from build123d import *

# Parameters (mm, degrees)
F0_R          = 3.85802972
F2_DEPTH      = 3.81
F2_DEPTH_BACK = 3.81
F4_D          = 3.2004
F6_W          = 0.762
F6_H          = 4.191
F10_W         = 0.762
F10_H         = 4.191
F14_W         = 0.762
F14_H         = 4.191
F17_W         = 0.762
F17_H         = 4.191
F25_T1_DEPTH  = 17.6167754913
F25_T3_DEPTH  = 17.6167754913
F25_T5_DEPTH  = 17.6167754913
F25_T7_DEPTH  = 17.6167754913


# Not quite as in the source:
# - a fillet or chamfer that OpenCascade refuses, or shapes differently, is made with other operations: its cross-section is extruded or revolved along the edge and cut away or added


with BuildPart() as f2:
    # F0 (on Top) → F2 (new body, two sides)
    with BuildSketch(Plane.XY) as f2_sk:
        Circle(F0_R)
    extrude(amount=F2_DEPTH)
    extrude(f2_sk.sketch, amount=-F2_DEPTH_BACK)

    # F4 (through all)
    with Locations(Plane(origin=(0, 0, -3.81), x_dir=(1, 0, 0), z_dir=(0, 0, -1))):
        with Locations((0, 0)):
            Hole(F4_D / 2)

    # F6 (on offset) → F21 section 0
    with BuildSketch(Plane.YZ.offset(3.81)):
        Rectangle(F6_W, F6_H)
    # F20 (on offset) → F21 section 1
    with BuildSketch(Plane.YZ.offset(15.24)):
        Polygon((-1.8273555028, -3.2485676474), (-1.0653555028, -3.2485676474), (1.8273555028, 3.2485676474), (1.0653555028, 3.2485676474), align=None)
    loft()

    # F10 (on offset) → F22 section 0
    with BuildSketch(Plane.XZ.offset(-3.81)):
        Rectangle(F10_W, F10_H)
    # F11 (on offset) → F22 section 1
    with BuildSketch(Plane.XZ.offset(-15.24)):
        Polygon((-1.8273555028, 3.2485676474), (1.0653555028, -3.2485676474), (1.8273555028, -3.2485676474), (-1.0653555028, 3.2485676474), align=None)
    loft()

    # F14 (on offset) → F23 section 0
    with BuildSketch(Plane.YZ.offset(-3.81)):
        Rectangle(F14_W, F14_H)
    # F19 (on offset) → F23 section 1
    with BuildSketch(Plane.YZ.offset(-15.24)):
        Polygon((1.0653555028, -3.2485676474), (1.8273555028, -3.2485676474), (-1.0653555028, 3.2485676474), (-1.8273555028, 3.2485676474), align=None)
    loft()

    # F17 (on offset) → F24 section 0
    with BuildSketch(Plane.XZ.offset(3.81)):
        Rectangle(F17_W, F17_H)
    # F18 (on offset) → F24 section 1
    with BuildSketch(Plane.XZ.offset(15.24)):
        Polygon((-1.8273555028, -3.2485676474), (-1.0653555028, -3.2485676474), (1.8273555028, 3.2485676474), (1.0653555028, 3.2485676474), align=None)
    loft()

    # F25: fillet of radius 3.048 on 8 edges, made by hand

    # F25_s2 → F25_t1 (cut)
    with BuildSketch(Plane.XZ.offset(-7.3620322429)):
        with BuildLine():
            ThreePointArc((-11.8860680784, 2.9102202816), (-14.2362386728, 2.1384513865), (-15.24, -0.1223874509))
            Line((-15.24, -0.1223874509), (-15.24, 3.2485676474))
            Line((-15.24, 3.2485676474), (-11.8860680784, 2.9102202816))
        make_face()
        with BuildLine():
            ThreePointArc((11.8860680784, -2.9102202816), (14.2362386728, -2.1384513865), (15.24, 0.1223874509))
            Line((15.24, 0.1223874509), (15.24, -3.2485676474))
            Line((15.24, -3.2485676474), (11.8860680784, -2.9102202816))
        make_face()
    extrude(amount=F25_T1_DEPTH, mode=Mode.SUBTRACT)

    # F25_s4 → F25_t3 (cut)
    with BuildSketch(Plane.XZ.offset(-10.2547432484)):
        with BuildLine():
            ThreePointArc((-11.8860680784, -2.9102202816), (-14.2362386728, -2.1384513865), (-15.24, 0.1223874509))
            Line((-15.24, 0.1223874509), (-15.24, -3.2485676474))
            Line((-15.24, -3.2485676474), (-11.8860680784, -2.9102202816))
        make_face()
        with BuildLine():
            ThreePointArc((11.8860680784, 2.9102202816), (14.2362386728, 2.1384513865), (15.24, -0.1223874509))
            Line((15.24, -0.1223874509), (15.24, 3.2485676474))
            Line((15.24, 3.2485676474), (11.8860680784, 2.9102202816))
        make_face()
    extrude(amount=F25_T3_DEPTH, mode=Mode.SUBTRACT)

    # F25_s6 → F25_t5 (cut)
    with BuildSketch(Plane.YZ.offset(-7.3620322429)):
        with BuildLine():
            ThreePointArc((11.8860680784, -2.9102202816), (14.2362386728, -2.1384513865), (15.24, 0.1223874509))
            Line((15.24, 0.1223874509), (15.24, -3.2485676474))
            Line((15.24, -3.2485676474), (11.8860680784, -2.9102202816))
        make_face()
        with BuildLine():
            ThreePointArc((-11.8860680784, 2.9102202816), (-14.2362386728, 2.1384513865), (-15.24, -0.1223874509))
            Line((-15.24, -0.1223874509), (-15.24, 3.2485676474))
            Line((-15.24, 3.2485676474), (-11.8860680784, 2.9102202816))
        make_face()
    extrude(amount=F25_T5_DEPTH, mode=Mode.SUBTRACT)

    # F25_s8 → F25_t7 (cut)
    with BuildSketch(Plane.YZ.offset(-10.2547432484)):
        with BuildLine():
            ThreePointArc((11.8860680784, 2.9102202816), (14.2362386728, 2.1384513865), (15.24, -0.1223874509))
            Line((15.24, -0.1223874509), (15.24, 3.2485676474))
            Line((15.24, 3.2485676474), (11.8860680784, 2.9102202816))
        make_face()
        with BuildLine():
            ThreePointArc((-11.8860680784, -2.9102202816), (-14.2362386728, -2.1384513865), (-15.24, 0.1223874509))
            Line((-15.24, 0.1223874509), (-15.24, -3.2485676474))
            Line((-15.24, -3.2485676474), (-11.8860680784, -2.9102202816))
        make_face()
    extrude(amount=F25_T7_DEPTH, mode=Mode.SUBTRACT)


solid = f2.part
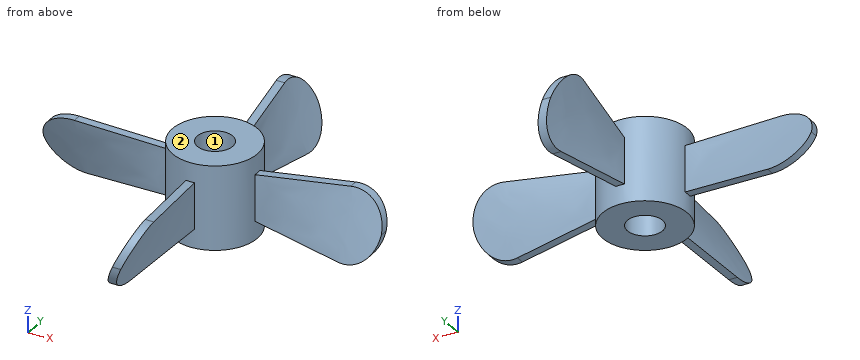
Part model, mm, in its own coordinate system. Face numbers are marked on the shaded views. Coordinates: 2 decimals unless noted, no trailing zeros. Use a Markdown table: item, result. Add a question column.
Item 1: Flat gauge pins, fed straight in: P1, Ø2, axis at y = 11.5, z = 1.5, coming from the -X side; P2, Ø4, axis at x = 5, z = -3, coming from the -Y side; P3, Ø2, axis at x = -9.5, z = 0, coming from the -Y side. Where does each tip first touch, or does it go through?
Item 2: Probe probe 1 along Y at (x, z) = (0, -3.5); probe 2 along X at (y, z) = (-9.5, 0); probe 3 along Y at (x, z) = (-1, 0.5). List the from-to ranges inside material, lowest first.
Item 3: Pull direction X, two halves, no side cores. Call the marked faces 1 and 2: +X half, -X half, draft (parallel to the pull), parting line (faces both ways), or undercut.
Geometry says:
| question | item | result |
|---|---|---|
| 1 | P1 | x = -1.24 |
| 1 | P2 | y = -2.43 |
| 1 | P3 | y = -0.65 |
| 2 | probe 1 | -3.86 to -1.6, 1.6 to 3.86 |
| 2 | probe 2 | -0.38 to 0.38 |
| 2 | probe 3 | -3.73 to -1.25, 1.25 to 3.73 |
| 3 | face 1 | undercut |
| 3 | face 2 | draft |
